```python
from build123d import *

# Parameters (mm, degrees)
F_6_0_6_DIAMETER_HOLE1_D     = 6
F_6_0_6_DIAMETER_HOLE1_DEPTH = 20
F_6_0_6_DIAMETER_HOLE1_TIP   = 1.802581857
SKETCH16_R                   = 1.5
CUT_EXTRUDE5_DEPTH           = 26


with BuildPart() as part:
    # Sketch3 → Revolve1 (revolve)
    with BuildSketch(Plane.XY):
        Polygon((0, 0), (4, 0), (5, 1), (5, 25), (0, 25), align=None)
    revolve(axis=Axis((0, 31.444228921, 0), (0, -1, 0)))

    # Ø6.0 (6) Diameter Hole1
    with Locations(Plane(origin=(0, 25, 0), x_dir=(1, 0, 0), z_dir=(0, 1, 0))):
        with Locations((0, 0)):
            Hole(F_6_0_6_DIAMETER_HOLE1_D / 2, depth=F_6_0_6_DIAMETER_HOLE1_DEPTH)
            with Locations((0, 0, -(F_6_0_6_DIAMETER_HOLE1_DEPTH + F_6_0_6_DIAMETER_HOLE1_TIP / 2))):  # 118° drill point
                Cone(0, F_6_0_6_DIAMETER_HOLE1_D / 2, F_6_0_6_DIAMETER_HOLE1_TIP, mode=Mode.SUBTRACT)

    # Sketch16 → Cut-Extrude5 (cut, through all)
    with BuildSketch(Plane(origin=(0, 25, 0), x_dir=(1, 0, 0), z_dir=(0, 1, 0))):
        Circle(SKETCH16_R)
    extrude(amount=-CUT_EXTRUDE5_DEPTH, mode=Mode.SUBTRACT)


solid = part.part
```
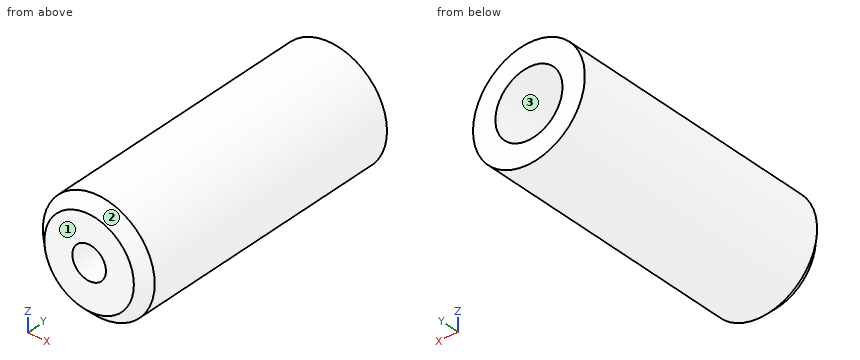
Can you work these out from the model? Positions are in its coordinate system, mm. Face numbers are marked on the shaded views. Give positions to 0.01 mm unless a question says otherwise; leave off trailing zeros. Loops run counter-clockwise (first coordinate to the right, second up) from the corner with the lowest first, then second, coordinate; pieces in that order, holes last. Notation, with made-up numbers: M 18.5,48.5 L 63.5,48.5 A30 ccw 63.5,81.5 Z; hole C 15.25,-24 d11. An arc over 180 degrees is marked long. One line per item, written item: value.
(1) Suppose I cut it at A-A on x = 0. List the corners of the cut face in (y, z) for me.
Returned:
outline: M 0,-4 L 1,-5 L 25,-5 L 25,-3 L 5,-3 L 4.1,-1.5 L 0,-1.5 Z; M 0,1.5 L 4.1,1.5 L 5,3 L 25,3 L 25,5 L 1,5 L 0,4 Z
(2) We'd pull the mould along Z, two halves only. Please class the marked faces 1, 2 and 3: released by +Z, released by -Z, zero draft, split by the parting line, or undercut.
Returned:
face 1: zero draft
face 2: split by the parting line
face 3: undercut
(3) Suppose I cut it at B-B on z = 0. List the corners of the cut face in (x, y) for me.
Returned:
outline: M -5,1 L -4,0 L -1.5,0 L -1.5,4.1 L -3,5 L -3,25 L -5,25 Z; M 1.5,0 L 4,0 L 5,1 L 5,25 L 3,25 L 3,5 L 1.5,4.1 Z
(4) Suppose I cut it at C-C on y = 10.25. List the corners of the cut face in (x, z) for me, plus the area to 3 significant figures.
Returned:
outline: C 0,0 d10; hole C 0,0 d6
area: 50.3 mm^2
(5) I need wall thicknesses on line 1 (Z direction, x = 0, y = 2); line 2 (Z direction, x = 2.25, y = 12.5); line 3 (X direction, y = 3, z = 3). Which ranges of each line are inside material? Lowest first, please.
Returned:
line 1: -5 to -1.5, 1.5 to 5
line 2: -4.47 to -1.98, 1.98 to 4.47
line 3: -4 to 4
(6) Will these pins go through, and if not, where does the flat tip stop? pin 1 (2.5 mm diameter, centred on x = 0, z = 0, fed in from -Y); pin 2 (1 mm diameter, centred on x = -1.5, y = 18, fed in from +Z); pin 3 (1.5 mm diameter, centred on x = -4, y = 22, fed in from -Z); pin 4 (1 mm diameter, centred on x = 1.5, y = 12.5, fed in from -Z).
Returned:
pin 1: through
pin 2: z = 4.9
pin 3: z = -3.8
pin 4: z = -4.9
